```python
from build123d import *

# Parameters (mm, degrees)
F2_DEPTH = 25.4
F3_F1_R  = 5.08
F3_F2_R  = 5.08
F6_D     = 6.35


# Not quite as in the source:
# - the program builds the solid bodies; features that only make, move or delete a surface that nothing else refers to are left out


with BuildPart() as f2:
    # F1 (on Top) → F2 (new body)
    with BuildSketch(Plane.XY):
        Polygon((-107.0532500744, -79.1042298079), (0, -35.2327227592), (107.0532500744, -79.1042298079), (55.5592626333, -19.3102359772), (46.5817004442, 0), (55.5592626333, 19.3102359772), (107.0532500744, 79.1042298079), (0, 35.2327227592), (-107.0532500744, 79.1042298079), (-55.5592626333, 19.3102359772), (-46.5817004442, 0), (-55.5592626333, -19.3102359772), align=None)
    extrude(amount=F2_DEPTH)

    # F3: fillet of radius 5.08 on 32 edges, made by hand

    # F3_f1
    f3_f1_edges = [f2.edges().sort_by_distance(p)[0] for p in [
        (-55.5592626333, -19.3102359772, 12.7),
        (-46.5817004442, 0, 12.7),
        (-55.5592626333, 19.3102359772, 12.7),
        (55.5592626333, -19.3102359772, 12.7),
        (46.5817004442, 0, 12.7),
        (55.5592626333, 19.3102359772, 12.7),
    ]]
    fillet(f3_f1_edges, radius=F3_F1_R)

    # F3_f2
    f3_f2_edges = [f2.edges().sort_by_distance(p)[0] for p in [
        (53.5266250372, 57.1684762836, 25.4),
        (53.5266250372, 57.1684762836, 0),
        (107.0532500744, 79.1042298079, 12.7),
        (81.5362590314, 49.4743083195, 25.4),
        (51.4197227557, 10.4063163842, 25.4),
        (51.4197227557, -10.4063163842, 25.4),
        (81.5362590314, -49.4743083195, 25.4),
        (107.0532500744, -79.1042298079, 12.7),
        (53.5266250372, -57.1684762836, 0),
        (53.5266250372, -57.1684762836, 25.4),
        (-81.5362590314, 49.4743083195, 25.4),
        (-53.5266250372, 57.1684762836, 25.4),
        (-51.4197227557, 10.4063163842, 25.4),
        (-51.4197227557, -10.4063163842, 25.4),
        (-81.5362590314, -49.4743083195, 25.4),
        (-53.5266250372, 57.1684762836, 0),
        (-107.0532500744, 79.1042298079, 12.7),
        (-81.5362590314, 49.4743083195, 0),
        (-53.5266250372, -57.1684762836, 0),
        (-107.0532500744, -79.1042298079, 12.7),
        (-53.5266250372, -57.1684762836, 25.4),
        (81.5362590314, -49.4743083195, 0),
        (51.4197227557, -10.4063163842, 0),
        (51.4197227557, 10.4063163842, 0),
        (-51.4197227557, 10.4063163842, 0),
        (-51.4197227557, -10.4063163842, 0),
        (-47.1038678133, 0, 0),
        (-55.6001625442, -19.2838429205, 0),
        (-55.6001625442, 19.2838429205, 0),
        (47.1038678133, 0, 0),
        (55.6001625442, 19.2838429205, 0),
        (55.6001625442, -19.2838429205, 0),
        (-55.6001625442, -19.2838429205, 25.4),
        (-47.1038678133, 0, 25.4),
        (-55.6001625442, 19.2838429205, 25.4),
        (55.6001625442, -19.2838429205, 25.4),
        (47.1038678133, 0, 25.4),
        (55.6001625442, 19.2838429205, 25.4),
    ]]
    fillet(f3_f2_edges, radius=F3_F2_R)

    # F6 (through all)
    with Locations(Plane.XY.offset(25.4)):
        with Locations((0, 0)):
            Hole(F6_D / 2)


solid = f2.part
```
The listing builds one solid part. Answer for the finished solid, in the listing's coordinates (mm). A direction names the side the tool comes from. Give positions to 0.01 mm unless a question says otherwise; leave off trailing zeros. Loops run counter-clockwise (first coordinate to the right, second up) from the corner with the lowest first, then second, coordinate; pieces in that order, holes last. Notation, with made-up numbers: (-12.75, -17) - (30.25, -17) arc R21 ccw to (30.25, -10) - close; hole circle Ø9 at (54, 64.5). An arc over 180 degrees is marked (long way). Return JSON: item names as keys, results as strings. Group by question number.
1. Determine the mould class of faces 1 (the cylindrical face through (43.97, -51.6, 1.45)), 2 (the flat face through (-74.888, 41.754, 12.593)), 3 (the flat face through (-1, 16, 0)) for opening direction Y: pulls with the +Y half, pulls with the -Y half, needs draft (parallel to the pull), parting line crosses it, or undercut.
2. Straight lines are drawn through the part: line 1 (X direction, y = 0.5, z = 8); line 2 (Z direction, x = -60.5, y = 55); line 3 (Y direction, x = -75.5, z = 11.5). For each, find the intervals that lie inside material, in ascending order. Write a range as [from, to].
3. Given pin 1 Ø5 at (x, y) = (-26, 46.5) entering from +Z; pin 2 Ø10 at (x, y) = (69.5, -21) entering from +Z; pin 3 Ø8 at (x, y) = (-36.5, 50.5) entering from -Z; pin 4 Ø4 at (x, y) = (-20, -44) entering from -Z, each flat-ended and moving along its own axis, determine where each tip first touches the part or whether it passes through.
4. Find section A-A (y = 0). Write down the section's boundary in (x, z) (3 decimals).
5. Find section B-B (z = 23.25). Write down the section's boundary in (x, y) (3 decimals), then the cut area to 3 significant figures.
6. Which of the six approach directions +Z, -Z, +X, -X, +Y, -Y give full straight-line access (tool end or side, diameter ignored) to faces 4 (the flat face through (51.474, -10.522, 12.593)), 5 (the flat face through (-74.37, -41.15, 12.59)), 6 (the cylindrical face through (-73.209, 42.146, 23.951))?
7. Find section C-C (z = 9.5). Write down the section's boundary in (x, y) (3 decimals).
Verdict:
{
 "1": {"face 1": "pulls with the -Y half", "face 2": "undercut", "face 3": "needs draft"},
 "2": {"line 1": "x = [-47.13, -3.14], [3.14, 47.13]", "line 2": "z = [0.02, 25.38]", "line 3": "y = [-66.17, -42.47], [42.47, 66.17]"},
 "3": {"pin 1": "stops at z = 24.31", "pin 2": "passes through", "pin 3": "stops at z = 0.19", "pin 4": "stops at z = 1.5"},
 "4": {"outline": "(-47.104, 5.08) arc R5.08 ccw to (-42.024, 0) - (-3.175, 0) - (-3.175, 25.4) - (-42.024, 25.4) arc R5.08 ccw to (-47.104, 20.32) - close; (3.175, 0) - (42.024, 0) arc R5.08 ccw to (47.104, 5.08) - (47.104, 20.32) arc R5.08 ccw to (42.024, 25.4) - (3.175, 25.4) - close"},
 "5": {"outline": "(-92.53, -63.666) arc R4.15 ccw to (-87.812, -70.214) - (0, -34.228) - (87.812, -70.214) arc R4.15 ccw to (92.53, -63.666) - (55.314, -20.451) arc R6.01 cw to (54.419, -19.063) - (46.734, -2.534) arc R6.01 cw to (46.734, 2.534) - (54.419, 19.063) arc R6.01 cw to (55.314, 20.451) - (92.53, 63.666) arc R4.15 ccw to (87.812, 70.214) - (0, 34.228) - (-87.812, 70.214) arc R4.15 ccw to (-92.53, 63.666) - (-55.314, 20.451) arc R6.01 cw to (-54.419, 19.063) - (-46.734, 2.534) arc R6.01 cw to (-46.734, -2.534) - (-54.419, -19.063) arc R6.01 cw to (-55.314, -20.451) - close; hole circle Ø6.35 at (0, 0)", "area": "13,000 mm^2"},
 "6": {"face 4": "+Z, -Z, +X", "face 5": "+Z, -Z, -X", "face 6": "+Z, -X"},
 "7": {"outline": "(-93.235, -63.059) arc R5.08 ccw to (-87.46, -71.075) - (0, -35.233) - (87.46, -71.075) arc R5.08 ccw to (93.235, -63.059) - (56.019, -19.844) arc R5.08 cw to (55.262, -18.671) - (47.577, -2.142) arc R5.08 cw to (47.577, 2.142) - (55.262, 18.671) arc R5.08 cw to (56.019, 19.844) - (93.235, 63.059) arc R5.08 ccw to (87.46, 71.075) - (0, 35.233) - (-87.46, 71.075) arc R5.08 ccw to (-93.235, 63.059) - (-56.019, 19.844) arc R5.08 cw to (-55.262, 18.671) - (-47.577, 2.142) arc R5.08 cw to (-47.577, -2.142) - (-55.262, -18.671) arc R5.08 cw to (-56.019, -19.844) - close; hole circle Ø6.35 at (0, 0)"}
}
